For this review, take the finished solid that the model builds, in its own axes (mm). A direction names the side the tool comes from. Give positions to 0.01 mm unless a question says otherwise; leave off trailing zeros. Order: outer loops, then holes, each group sorted by start corner. A loop starts at its lowest first (then second) coordinate and runs counter-clockwise, first axis right, second up.
Item 1: Machinability: for faces 1 (the flat face through (-7, 34.069, 49)), 2 (the flat face through (-7, -28.174, 74)), which of the approach directions +Z, -Z, +X, -X, +Y, -Y give a long, thin tool a straight path to every point of the face, cutting with its end or side? Answer none if there is none.
Item 2: For P1, Ø4, axis at x = 17, y = -24.5, coming from the -Z side; P2, Ø14, axis at x = -20, z = 71, coming from the -Y side, all flat-tipped, find the tip position at first contact; note any pin that passes through.
Item 3: For probe 1 along Y at (x, z) = (-48.5, 90.5), list the stretches that pass through material, from the lowest coordinate up.
Item 4: Consider section B-B (z = 79). Give the boundary of the cut face in (x, y), plus the area to 3 significant figures.
Item 5: Consider section A-A (x = -31). Give the boundary of the cut face in (y, z), plus the area to 3 significant figures.
```python
from build123d import *

# Parameters (mm, degrees)
F0_W      = 97.864177
F0_H      = 67.323104
F1_DEPTH  = 51.054
F2_R      = 5.08
F1_FACE_W = 97.864178
F1_FACE_H = 62.243104
F3_DEPTH  = 47.498


with BuildPart() as f1:
    # F0 (on Top) → F1 (new body)
    with BuildSketch(Plane.XY):
        with Locations((-6.312856, 0.407133)):
            Rectangle(F0_W, F0_H)
    extrude(amount=F1_DEPTH)

    # F2
    f2_edges = [f1.edges().sort_by_distance(p)[0] for p in [
        (-6.312856, -33.254419, 51.054),
    ]]
    fillet(f2_edges, radius=F2_R)

    # F1_face (on face) → F3 (join)
    with BuildSketch(Plane(origin=(-6.312856, 2.947133, 51.054), x_dir=(1, 0, 0), z_dir=(0, 0, 1))):
        Rectangle(F1_FACE_W, F1_FACE_H)
    extrude(amount=F3_DEPTH)


solid = f1.part
```
Resolved:
1. face 1: +Z, -Z, +X, -X, +Y
1. face 2: +Z, +X, -X, -Y
2. P1: stops at z = 0
2. P2: stops at y = -28.17
3. probe 1: y = -28.17 to 34.07
4. outline: (-55.24, -28.17) - (42.62, -28.17) - (42.62, 34.07) - (-55.24, 34.07) - close
4. area: 6,090 mm2
5. outline: (-33.25, 0) - (34.07, 0) - (34.07, 98.55) - (-28.17, 98.55) - (-28.17, 51.05) arc R5.08 ccw to (-33.25, 45.97) - close
5. area: 6,390 mm2
